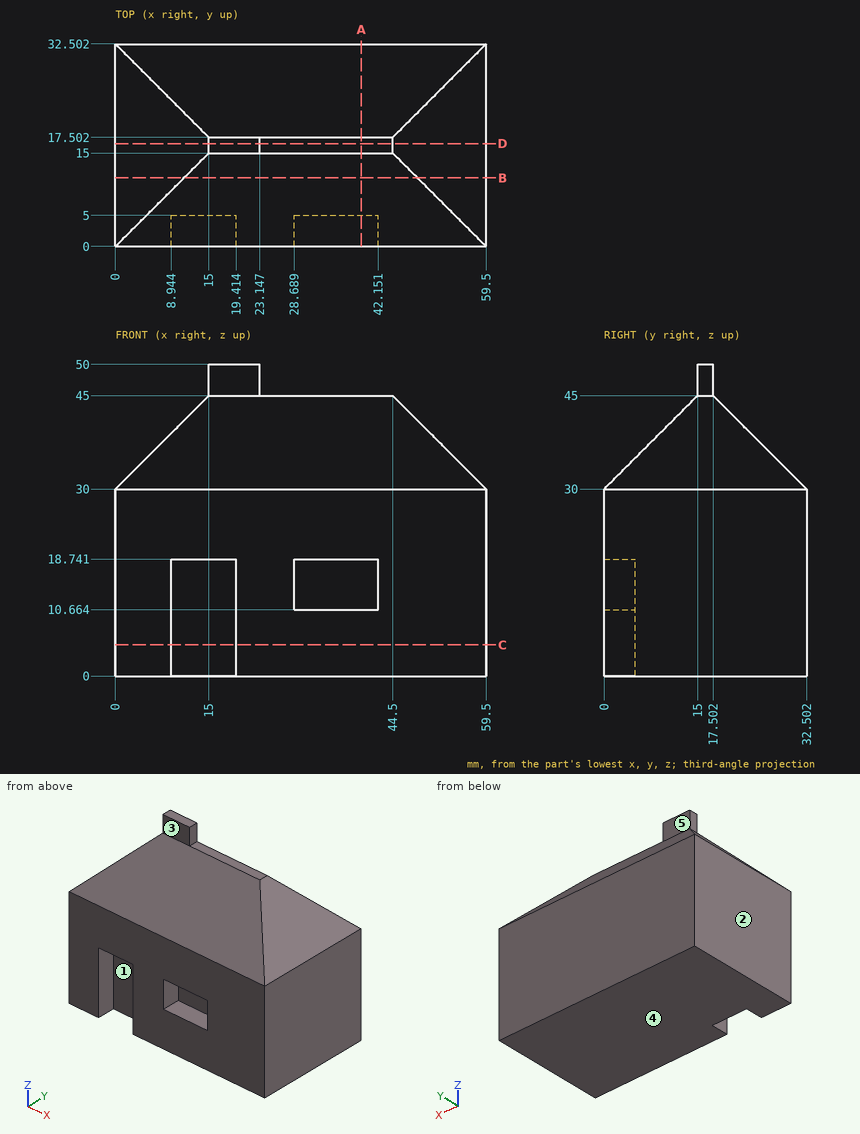
Here's the drawing with two shaded views (mm, measured from the low corner). I have some questions. A direction names the side the tool comes from. Coordinates: 2 decimals unless noted, no trailing zeros. Loops run counter-clockwise (first coordinate to the right, second up) from the corner with the lowest first, then second, coordinate; pieces in that order, holes last. Notation, with made-up numbers: (28, -8) -> (81, -8) arc R31 cw to (81, 31) -> close; hole circle Ø10 at (23.5, -36). An arc over 180 degrees is marked (long way). Answer as a JSON object with one key per item and string values.
1) If I drill on line 1 (X direction, y = 2.5, z = 8.5) (1 decimal); line 2 (Y direction, x = 16.5, z = 47); line 3 (Y direction, x = 39, z = 13), over which ranges is the centre line in solid material (lowest first)?
Results:
{"line 1": "x = 0 to 8.9, 19.4 to 59.5", "line 2": "y = 15 to 17.5", "line 3": "y = 5 to 32.5"}
2) Imagine slicing it at A-A (x = 39.5). Please give me the cut outline in (y, z) (1 decimal), then the cut area to 3 significant figures.
Results:
{"outline": "(0, 0) -> (32.5, 0) -> (32.5, 30) -> (17.5, 45) -> (15, 45) -> (0, 30) -> (0, 18.7) -> (5, 18.7) -> (5, 10.7) -> (0, 10.7) -> close", "area": "1,200 mm^2"}
3) For the marked faces 4 and 5, which set-ups out of +Z, -Z, +X, -X, +Y, -Y let a thin tool reach every point of the face, with its end or its side?
Results:
{"face 4": "-Z, +X, -X, +Y, -Y", "face 5": "+Z, +X, -X, +Y"}
4) Thinking about a two-plate mould opening in X: for the marked faces 1, 2 and 3, which applies, pulls with the +X half, pulls with the -X half, needs draft (parallel to the pull), parting line crosses it, or undercut?
Results:
{"face 1": "undercut", "face 2": "pulls with the -X half", "face 3": "needs draft"}
5) For P1, Ø3, axis at x = 25, y = 12.5, coming from the +Z side; P2, Ø1.5, axis at x = 15.5, y = 2, coming from the -Z side; P3, Ø1.5, axis at x = 14.5, y = 11, coming from the +Z side, each with a flat end and sliding along its axis, tell me the tip position at first contact or that it passes through.
Results:
{"P1": "stops at z = 44", "P2": "stops at z = 18.74", "P3": "stops at z = 41.75"}
6) Imagine slicing it at C-C (z = 5). Please give me the cut outline in (x, y) (1 decimal).
Results:
{"outline": "(0, 0) -> (8.9, 0) -> (8.9, 5) -> (19.4, 5) -> (19.4, 0) -> (59.5, 0) -> (59.5, 32.5) -> (0, 32.5) -> close"}
7) Imagine slicing it at D-D (y = 16.5). Please give me the cut outline in (x, z).
Results:
{"outline": "(0, 0) -> (59.5, 0) -> (59.5, 30) -> (44.5, 45) -> (23.15, 45) -> (23.15, 50) -> (15, 50) -> (15, 45) -> (0, 30) -> close"}
8) Imagine slicing it at B-B (y = 11). Please give me the cut outline in (x, z).
Results:
{"outline": "(0, 0) -> (59.5, 0) -> (59.5, 30) -> (48.5, 41) -> (11, 41) -> (0, 30) -> close"}
